from build123d import *

# Parameters (mm, degrees)
SKETCH_1_W      = 45
SKETCH_1_H      = 8
SKETCH_1_R      = 1
EXTRUDE_1_DEPTH = 1.2
SKETCH_3_W      = 45
SKETCH_3_H      = 1.2
EXTRUDE_2_DEPTH = 7


with BuildPart() as part:
    # ｽｹｯﾁ1 → ﾎﾞｽ - 押し出し1 (new body)
    with BuildSketch(Plane(origin=(0, 0, 0), x_dir=(0, 1, 0), z_dir=(0, 0, 1))):
        with Locations((22.5, 4)):
            Rectangle(SKETCH_1_W, SKETCH_1_H)
        with Locations(Location((2.3, 4, 0), (0, 0, 270))):
            Circle(SKETCH_1_R, mode=Mode.SUBTRACT)
        with Locations(Location((42.7, 4, 0), (0, 0, 90))):
            Circle(SKETCH_1_R, mode=Mode.SUBTRACT)
    extrude(amount=-EXTRUDE_1_DEPTH)

    # ｽｹｯﾁ3 → ﾎﾞｽ - 押し出し2 (add)
    with BuildSketch(Plane(origin=(-8, 0, 0), x_dir=(0, -1, 0), z_dir=(-1, 0, 0))):
        with Locations((-22.5, -0.6)):
            Rectangle(SKETCH_3_W, SKETCH_3_H)
    extrude(amount=EXTRUDE_2_DEPTH)


solid = part.part
Read the model definition and answer for the solid it produces. Units are mm, in the model's axes. Round coordinates to 2 decimals unless told otherwise and drop trailing zeros. Write each loop counter-clockwise with the first axis right and the second up, starting at its lowest first coordinate (ties: lowest second). Pieces come first, ordered by that corner, then holes. Notation, with made-up numbers: M 30,-25 L 88,-25 A26 ccw 88,7 Z; hole C 33,66.25 d6. An arc over 180 degrees is marked long. Use a Markdown table: item, result.
1) Straight lines are drawn through the part: line 1 along Y through (x, z) = (-4, -0.45); line 2 along X through (y, z) = (42.7, -0.85). For each, find the intervals that lie inside material, in ascending order. Write a range as [from, to].
Answers follow:
| item | result |
|---|---|
| line 1 | y = [0, 1.3], [3.3, 41.7], [43.7, 45] |
| line 2 | x = [-15, -5], [-3, 0] |
2) A flat-ended cylindrical pin translates along its axis: pin 1 (1.2 mm diameter, centred on x = -4, y = 42.7, fed in from +Z). Find the tip coordinate at first contact, or state that the pin passes through.
Answers follow:
| item | result |
|---|---|
| pin 1 | passes through |
3) The part is cut by section B-B (x = -4). Write down the section's boundary in (y, z).
Answers follow:
| item | result |
|---|---|
| outline | M 0,-1.2 L 1.3,-1.2 L 1.3,0 L 0,0 Z; M 3.3,-1.2 L 41.7,-1.2 L 41.7,0 L 3.3,0 Z; M 43.7,-1.2 L 45,-1.2 L 45,0 L 43.7,0 Z |
4) For a pull along X with two mould halves and no side action, classify faces 1 (the cylindrical face through (-3.783, 43.676, -0.592)), 2 (the flat face through (0, 22, -1)), 3 (the flat face through (-7, 45, -1)), 4 (the cylindrical face through (-4.8, 1.7, -0.6)) as pulls with the +X half, pulls with the -X half, needs draft (parallel to the pull), parting line crosses it, or undercut.
Answers follow:
| item | result |
|---|---|
| face 1 | undercut |
| face 2 | pulls with the +X half |
| face 3 | needs draft |
| face 4 | undercut |
5) The part is cut by section A-A (y = 2.3). Write down the section's boundary in (x, z).
Answers follow:
| item | result |
|---|---|
| outline | M -15,-1.2 L -5,-1.2 L -5,0 L -15,0 Z; M -3,-1.2 L 0,-1.2 L 0,0 L -3,0 Z |
